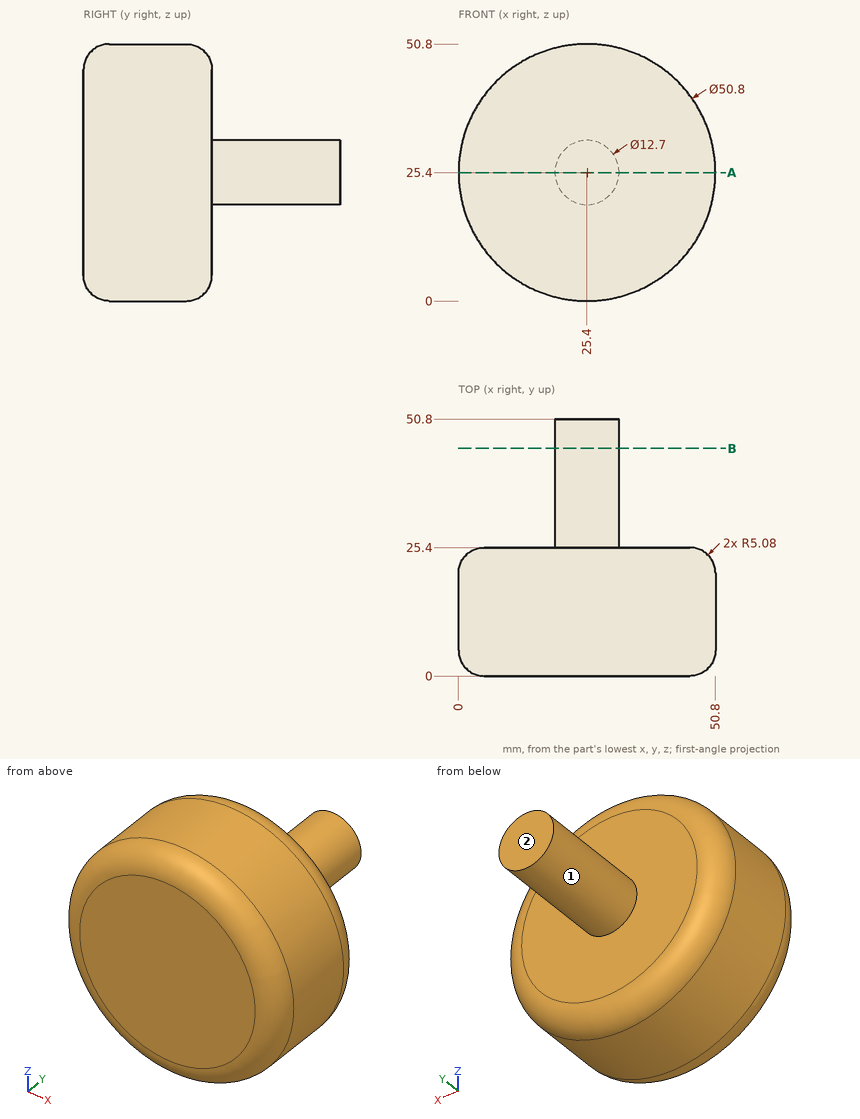
Part print with two shaded views. Sizes in mm from the minimum x, y, z corner. A direction names the side the tool comes from. Coordinates: 2 decimals unless noted, no trailing zeros. Order: outer loops, then holes, each group sorted by start corner. A loop starts at its lowest first (then second) coordinate and runs counter-clockwise, first axis right, second up.
(1) Drill centre lines: L1, parallel to Y at x = 25, z = 45; L2, parallel to X at y = 37, z = 26.5; L3, parallel to Z at x = 27, y = 3. Where is each one in solid material? Low to high.
Solution:
L1: y = 0 to 25.4
L2: x = 19.15 to 31.65
L3: z = 0.5 to 50.3
(2) Saw through at B-B, the plane y = 45. Write the cut outline in (x, z).
Solution:
outline: circle Ø12.7 at (25.4, 25.4)
(3) Which spindle directions (+Z, -Z, +X, -X, +Y, -Y) get a long thin tool onto all of the face, cutting with end or side? Do the marked faces 1 and 2. Say none if no direction does.
Solution:
face 1: +Y
face 2: +Z, -Z, +X, -X, +Y
(4) Pin check, flat tips, straight feed: pin 1 Ø1.5 at (x, y) = (32, 31.5) entering from +Z; pin 2 Ø1.5 at (y, z) = (24.5, 13.5) entering from +X; pin 3 Ø1 at (y, z) = (43, 19.5) entering from -X. Stop position of each tip, or through.
Solution:
pin 1: stops at z = 27.87
pin 2: stops at x = 46.42
pin 3: stops at x = 22.06
(5) Saw through at A-A, the plane z = 25.4. Write the cut outline in (x, y).
Solution:
outline: (0, 5.08) arc R5.08 ccw to (5.08, 0) - (45.72, 0) arc R5.08 ccw to (50.8, 5.08) - (50.8, 20.32) arc R5.08 ccw to (45.72, 25.4) - (31.75, 25.4) - (31.75, 50.8) - (19.05, 50.8) - (19.05, 25.4) - (5.08, 25.4) arc R5.08 ccw to (0, 20.32) - close
